The listing builds one solid part. Answer for the finished solid, in the listing's coordinates (mm). Face numbers are marked on the shaded views. A direction names the side the tool comes from. Give positions to 0.01 mm unless a question says otherwise; leave off trailing zeros. Loops run counter-clockwise (first coordinate to the right, second up) from the corner with the lowest first, then second, coordinate; pieces in that order, holes last.
Item 1: The mould has two halves that part along X. Classify the marked faces 3, 4 and 5: pulls with the +X half, pulls with the -X half, needs draft (parallel to the pull), parting line crosses it, or undercut.
Item 2: Section D-D, the plane z = -73.75 is taken. Give the vertices of the cut face in (x, y).
Item 3: Each of these flat-tipped pins is pushed along its axis until it touches: pin 1 Ø1.5 at (x, z) = (3.5, -78.5) entering from -Y; pin 2 Ø1.4 at (x, z) = (4, -76.5) entering from +Y. Where does it stop, or does it pass through?
Item 4: Section C-C, the plane y = 7.5 is taken. Give the vertices of the cut face in (x, z), and give its area (3 significant figures).
Item 5: A tool of negligible diameter and unlimited length cuts with its end or side. For the marked faces 1 and 2, from which of +Z, -Z, +X, -X, +Y, -Y can it reach the whole face along a straight path? Write none if from no direction.
Item 6: Section A-A, the plane z = -71 is taken. Give the vertices of the cut face in (x, y), and give its area (3 significant figures).
Item 7: Consider line 1 along Y through (x, z) = (3.5, -75.5); line 2 along Y through (x, z) = (6, -75); line 3 along Z through (x, y) = (-8.25, 27). Determine where each line is inside the solid, lowest interval first.
Item 8: Section B-B, the plane x = -2.5 is taken. Give the vertices of the cut face in (y, z).
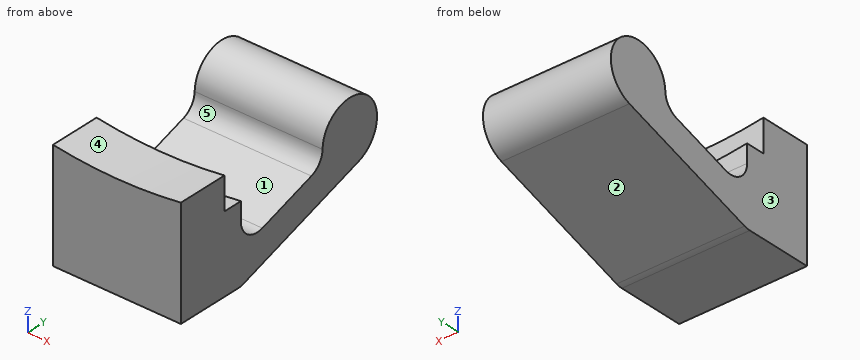
from build123d import *

# Parameters (mm, degrees)
BOSS_EXTRUDE1_DEPTH = 8
BOSS_EXTRUDE2_DEPTH = 3
BOSS_EXTRUDE3_DEPTH = 20
FILLET5_R           = 3


with BuildPart() as part:
    # Sketch1 → Boss-Extrude1 (new body)
    with BuildSketch(Plane(origin=(0, 0, 0), x_dir=(1, 0, 0), z_dir=(0, 1, 0))):
        with BuildLine():
            Line((-10, 69.282032303), (-10, 74.330343737))
            Line((-10, 74.330343737), (-10, 86.330343737))
            Line((-10, 86.330343737), (10, 86.330343737))
            Line((10, 86.330343737), (10, 74.330343737))
            Line((10, 74.330343737), (10, 69.282032303))
            ThreePointArc((10, 69.282032303), (0, 70), (-10, 69.282032303))
        make_face()
    extrude(amount=BOSS_EXTRUDE1_DEPTH)

    # Sketch2 → Boss-Extrude2 (add)
    with BuildSketch(Plane(origin=(0, 8, 0), x_dir=(1, 0, 0), z_dir=(0, 1, 0))):
        with BuildLine():
            Line((-10, 74.330343737), (-10, 86.330343737))
            Line((-10, 86.330343737), (10, 86.330343737))
            Line((10, 86.330343737), (10, 74.330343737))
            ThreePointArc((10, 74.330343737), (0, 75), (-10, 74.330343737))
        make_face()
    extrude(amount=BOSS_EXTRUDE2_DEPTH)

    # Sketch3 → Boss-Extrude3 (add)
    with BuildSketch(Plane(origin=(10, 0, 0), x_dir=(0, 0, -1), z_dir=(1, 0, 0))):
        with BuildLine():
            Line((81.330343737, 11), (86.330343737, 11))
            Line((86.330343737, 11), (79.069603203, 32.59355568))
            ThreePointArc((79.069603203, 32.59355568), (69.795873168, 33.106792981), (76.168874572, 26.350289862))
            Line((76.168874572, 26.350289862), (81.330343737, 11))
        make_face()
    extrude(amount=-BOSS_EXTRUDE3_DEPTH)

    # Fillet5
    fillet5_edges = [part.edges().sort_by_distance(p)[0] for p in [
        (0, 11, -86.330343737),
        (0, 11, -81.330343737),
        (0, 26.350289862, -76.168874572),
    ]]
    fillet(fillet5_edges, radius=FILLET5_R)


solid = part.part
Worked answers:
1. face 3: pulls with the -X half
1. face 4: undercut
1. face 5: needs draft
2. outline: (-10, 0) - (10, 0) - (10, 8) - (-10, 8) - close; (-10, 26.03) - (10, 26.03) - (10, 35.97) - (-10, 35.97) - close
3. pin 1: stops at y = 0
3. pin 2: stops at y = 35.78
4. outline: (-10, -86.33) - (10, -86.33) - (10, -69.28) arc R70 cw to (-10, -69.28) - close
4. area: 331 mm2
5. face 1: +Z, +X, -X
5. face 2: -Z, +X, -X, +Y
6. outline: (-10, 0) - (10, 0) - (10, 8) - (-10, 8) - close; (-10, 27.27) - (10, 27.27) - (10, 34.73) - (-10, 34.73) - close
6. area: 309 mm2
7. line 1: y = 0 to 11, 25.67 to 35.86
7. line 2: y = 0 to 11, 25.87 to 35.95
7. line 3: z = -80.95 to -71.33
8. outline: (0, -86.33) - (10.51, -86.33) arc R3 ccw to (11.47, -86.17) - (32.59, -79.07) arc R5 ccw (long way) to (26, -74.2) arc R3 cw to (23.96, -76.97) - (14.96, -80) arc R3 cw to (11, -77.16) - (11, -74.96) - (8, -74.96) - (8, -69.96) - (0, -69.96) - close
